Source: three-view drawing plus pictorial views. Frame: mm from the lowest corner of the part. Give positions to 0.01 mm unless a question says otherwise; leave off trailing zeros. Loops run counter-clockwise (first coordinate to the right, second up) from the corner with the lowest first, then second, coordinate; pieces in that order, holes last. Notation, with made-up numbers: (70, 42) - (88, 42) arc R8 ccw to (88, 56) - close; hole circle Ø11 at (69, 58). An arc over 180 degrees is marked (long way). Answer as a JSON object with one key per item and string values. Group by question number.
(1) Section query A-A (x = 13). Return loops of the section in (y, z), plus the area to 3 significant figures.
(2) Material intervals for L1, parallel to Y at x = 13, z = 2.35; L2, parallel to Y at x = 36, z = 1.6; L3, parallel to X at y = 9.5, z = 1.75, sorted ascending.
(3) Section query B-B (y = 11). Return loops of the section in (x, z), plus the area to 3 significant figures.
(4) Pin query (flat end, axial travel): P1, Ø1, axis at x = 15.5, y = 6, coming from the -Z side; P2, Ø2.5, axis at x = 13, y = 29, coming from the -Z side. Return the tip coordinate at first contact, or that it passes through.
(5) Section query C-C (z = 1.05). Return loops of the section in (x, y), plus the area to 3 significant figures.
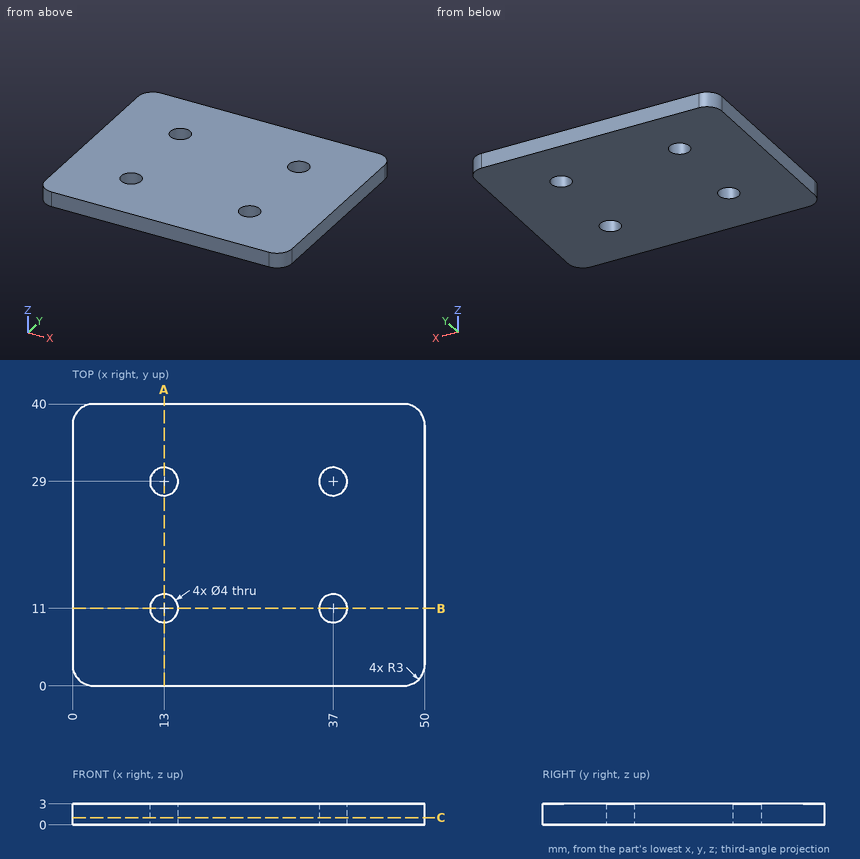
Recorded:
{
 "1": {"outline": "(0, 0) - (9, 0) - (9, 3) - (0, 3) - close; (13, 0) - (27, 0) - (27, 3) - (13, 3) - close; (31, 0) - (40, 0) - (40, 3) - (31, 3) - close", "area": "96.0 mm^2"},
 "2": {"L1": "y = 0 to 9, 13 to 27, 31 to 40", "L2": "y = 0 to 9.27, 12.73 to 27.27, 30.73 to 40", "L3": "x = 0 to 11.68, 14.32 to 35.68, 38.32 to 50"},
 "3": {"outline": "(0, 0) - (11, 0) - (11, 3) - (0, 3) - close; (15, 0) - (35, 0) - (35, 3) - (15, 3) - close; (39, 0) - (50, 0) - (50, 3) - (39, 3) - close", "area": "126 mm^2"},
 "4": {"P1": "stops at z = 0", "P2": "passes through"},
 "5": {"outline": "(0, 3) arc R3 ccw to (3, 0) - (47, 0) arc R3 ccw to (50, 3) - (50, 37) arc R3 ccw to (47, 40) - (3, 40) arc R3 ccw to (0, 37) - close; hole circle Ø4 at (13, 11); hole circle Ø4 at (13, 29); hole circle Ø4 at (37, 11); hole circle Ø4 at (37, 29)", "area": "1,940 mm^2"}
}
